The model under review builds one solid part; all positions refer to its coordinate system, in mm. A direction names the side the tool comes from. Round coordinates to 2 decimals unless told otherwise and drop trailing zeros. Loops run counter-clockwise (first coordinate to the right, second up) from the corner with the lowest first, then second, coordinate; pieces in that order, holes last. Notation, with made-up numbers: M 69.5,57 L 126.5,57 A23 ccw 126.5,84 Z; hole C -24.75,16.5 d8. An arc over 180 degrees is marked long. Answer as a JSON object with one key per item and string values. Group by question number.
Item 1: To check wall thickness, follow line 1 (X direction, y = 20, z = 61.9); line 2 (Y direction, x = 16, z = 3.75); line 3 (X direction, y = -16, z = 6). State the ranges of each line that lie inside material, in increasing order.
Item 2: The part is to be moulded in two halves that separate along X. For faces 1 (the face through (-18, -16, 1.2)), 2 (the face through (0, 25, 62)), 3 (the face through (-23.889, 23.848, 64.658)), say which applies: +X half, -X half, draft (parallel to the pull), parting line (faces both ways), or undercut.
Item 3: Insertion check: P1, Ø1.5, axis at x = -3, y = 1.5, coming from the +Z side; P2, Ø3, axis at x = 3, z = 53, coming from the +Y side; P3, Ø12, axis at y = -2, z = 37.5, coming from the -X side. Each pin has a flat end and moves straight along its axis. Give the tip position at first contact, or say it passes through.
Item 4: Consider section B-B (z = 22). Give the boundary of the cut face in (x, y) (3 decimals).
Item 5: Tool access review of faces 4 (the face through (-0.189, 13.606, 3.944)), 5 (the face through (-8, 18, 10)), 6 (the face through (-0.189, -13.794, 4.056)), 7 (the face through (0.3, 20.4, 8.3)): name each direction out of +Z, -Z, +X, -X, +Y, -Y from which nothing blocks a thin tool from reaching the whole face with its end or side.
Solid Edge part; units mm, degrees
sketch "Sketch1" plane through (0, 0, 0) normal (0, 0, 1) x (1, 0, 0)
  line L0 (-21.4, -20.4) -> (21.4, -20.4)
  line L1 (21.4, -20.4) -> (21.4, 20.4)
  line L2 (21.4, 20.4) -> (-21.4, 20.4)
  line L3 (-21.4, 20.4) -> (-21.4, -20.4)
  circle A0 centre (0, 0) radius 4
extrude "Extrusionsausprägung_20" add sketch "Sketch1" along normal blind 10
sketch "Sketch2" plane through (0, 0, 0) normal (0, 0, -1) x (0, -1, 0)
  line L0 (19.55, 19.55) -> (12.45, 19.55)
  line L1 (12.45, 19.55) -> (12.45, 12.45)
  line L2 (12.45, 12.45) -> (19.55, 12.45)
  line L3 (19.55, 12.45) -> (19.55, 19.55)
extrude "Extrusionsausschnitt_24" cut sketch "Sketch2" against normal blind 1.2
hole "Bohrung_4" at (-16, -16, 0) direction (0, 0, 1) diameter 3.5 end up to next
mirror "Mirror1" about plane through (0, 0, 0) normal (0, -1, 0) of "Extrusionsausschnitt_24", "Bohrung_4"
mirror "Mirror2" about plane through (0, 0, 0) normal (1, 0, 0) of "Extrusionsausschnitt_24", "Bohrung_4", "Mirror1"
sketch "Sketch3" plane through (0, 0, 0) normal (1, 0, 0) x (0, 1, 0)
  line L0 (20.4, 0) -> (7, 0)
  line L1 (7, 0) -> (20.4, 8)
  line L2 (20.4, 8) -> (20.4, 0)
extrude "Extrusionsausschnitt_25" cut sketch "Sketch3" along normal mid plane 27
mirror "Mirror3" about plane through (0, 0, 0) normal (0, -1, 0) of "Extrusionsausschnitt_25"
sketch "Sketch4" plane through (0, 0, 10) normal (0, 0, 1) x (0, 1, 0)
  circle A0 centre (0, 0) radius 15.375
  circle A1 centre (0, 0) radius 17.5
extrude "Extrusionsausprägung_21" add sketch "Sketch4" along normal blind 54.8
chamfer "Fase_9" distance 2 angle 45 1 edges at (0, -17.5, 10)
sketch "Sketch5" plane through (0, 0, 64.8) normal (0, 0, 1) x (-1, 0, 0)
  line L0 (-25, 25) -> (-25, -25)
  line L1 (-25, -25) -> (25, -25)
  line L2 (25, -25) -> (25, 25)
  line L3 (25, 25) -> (-25, 25)
  circle A0 centre (0, 0) radius 15.375
extrude "Extrusionsausprägung_23" add sketch "Sketch5" against normal blind 5
chamfer "Fase_10" distance 3 angle 45 1 edges at (-17.5, 0, 59.8)
sketch "Sketch6" plane through (0, 0, 64.8) normal (0, 0, 1) x (0, -1, 0)
  circle A0 centre (-20, 20) radius 1.75
  circle A1 centre (-20, -20) radius 1.75
  circle A2 centre (20, -20) radius 1.75
  circle A3 centre (20, 20) radius 1.75
extrude "Extrusionsausschnitt_26" cut sketch "Sketch6" against normal blind 27
fillet "Verrundung_16" radius 3 4 edges at (-25, -25, 62.3) (25, -25, 62.3) (-25, 25, 62.3) (25, 25, 62.3)
chamfer "Fase_11" distance 0.5 angle 45 12 edges at (20, 21.75, 64.8) (-20, 21.75, 64.8) (-20, -18.25, 64.8) (20, -18.25, 64.8) (25, 0, 64.8) (24.1213, 24.1213, 64.8) (0, 25, 64.8) (-24.1213, 24.1213, 64.8) (-25, 0, 64.8) (-24.1213, -24.1213, 64.8) (0, -25, 64.8) (24.1213, -24.1213, 64.8)
chamfer "Fase_12" distance 1 angle 45 1 edges at (0, -15.375, 64.8)
Geometry results:
{
 "1": {"line 1": "x = -25 to -21.75, -18.25 to 18.25, 21.75 to 25", "line 2": "y = -20.4 to -17.75, -14.25 to 14.25, 17.75 to 20.4", "line 3": "x = -21.4 to -17.75, -14.25 to 14.25, 17.75 to 21.4"},
 "2": {"face 1": "undercut", "face 2": "draft", "face 3": "-X half"},
 "3": {"P1": "stops at z = 10", "P2": "stops at y = 17.44", "P3": "stops at x = -17.5"},
 "4": {"outline": "C 0,0 d35; hole C 0,0 d30.75"},
 "5": {"face 4": "-Z, +Y", "face 5": "none", "face 6": "-Z, -Y", "face 7": "-Z, +X, -X, +Y"}
}
